Here's how the part is built. I have some questions about the finished solid (model axes, mm). A direction names the side the tool comes from. Coordinates: 2 decimals unless noted, no trailing zeros. Order: outer loops, then holes, each group sorted by start corner. A loop starts at its lowest first (then second) coordinate and runs counter-clockwise, first axis right, second up.
```python
from build123d import *

# Parameters (mm, degrees)
F0_W     = 50.8
F0_H     = 38.1
F1_DEPTH = 12.7
F3_DEPTH = 12.7
F5_DEPTH = 12.7


with BuildPart() as f1:
    # F0 (on Front) → F1 (new body)
    with BuildSketch(Plane.XZ):
        with Locations((-46.846292, 55.045669)):
            Rectangle(F0_W, F0_H)
    extrude(amount=F1_DEPTH)

    # F2 (on face) → F3 (join)
    with BuildSketch(Plane.XZ.offset(12.7)):
        Polygon((-21.446292, 42.345669), (-72.246292, 55.045669), (-72.246292, 35.995669), (-21.446292, 35.995669), align=None)
    extrude(amount=F3_DEPTH)

    # F4 (on face) → F5 (join)
    with BuildSketch(Plane.XZ.offset(12.7)):
        Polygon((-34.146292, 74.095669), (-21.446292, 61.395669), (-21.446292, 74.095669), align=None)
    extrude(amount=F5_DEPTH)


solid = f1.part
```
Q1. I need wall thicknesses on L1, parallel to Y at x = -50.5, z = 54; L2, parallel to Z at x = -30.5, y = -20.5; L3, parallel to Z at x = -25.5, y = -15.5. Which ranges of each line are inside material? Lowest first, please.
Q2. If we section it at C-C on x = -55.5: Write out the boundary of the cut face in (y, z).
Q3. If we section it at B-B on z = 58: Write out the boundary of the cut face in (x, y).
Q4. Will this pin go through, and if not, where does the flat tip stop? pin 1 (2 mm diameter, centred on x = -38.5, z = 59, fed in from -Y).
Q5. For faces 1 (the flat face through (-27.885, -18.961, 67.835)), 2 (the flat face through (-47, -12.7, 62)), 3 (the flat face through (-46.491, -18.961, 48.607)), which set-ups out of +Z, -Z, +X, -X, +Y, -Y let a thin tool reach every point of the face, with its end or its side?
Q6. If we section it at D-D on z = 50: Write out the boundary of the cut face in (x, y), then the cut area to 3 significant figures.
Q7. If we section it at A-A on y = -19: Write out the boundary of the cut face in (x, z).
Reply:
1. L1: y = -12.7 to 0
1. L2: z = 36 to 44.61, 70.45 to 74.1
1. L3: z = 36 to 43.36, 65.45 to 74.1
2. outline: (-25.4, 36) - (0, 36) - (0, 74.1) - (-12.7, 74.1) - (-12.7, 50.86) - (-25.4, 50.86) - close
3. outline: (-72.25, -12.7) - (-21.45, -12.7) - (-21.45, 0) - (-72.25, 0) - close
4. pin 1: stops at y = -12.7
5. face 1: -X, -Y
5. face 2: -Y
5. face 3: +X, -Y
6. outline: (-72.25, -25.4) - (-52.06, -25.4) - (-52.06, -12.7) - (-21.45, -12.7) - (-21.45, 0) - (-72.25, 0) - close
6. area: 901 mm2
7. outline: (-72.25, 36) - (-21.45, 36) - (-21.45, 42.35) - (-72.25, 55.05) - close; (-34.15, 74.1) - (-21.45, 61.4) - (-21.45, 74.1) - close
